from build123d import *

# Parameters (mm, degrees)
SKETCH1_R           = 8.3185
BOSS_EXTRUDE1_DEPTH = 6.35
FILLET1_R           = 0.508
SHELL1_T            = -0.127
SKETCH11_W          = 13.94567027
SKETCH11_H          = 5.377156333
CUT_EXTRUDE1_DEPTH  = 9.144
BOSS_EXTRUDE2_DEPTH = 1.27
SKETCH14_R          = 2.413
SKETCH14_R_2        = 2.316819153
CUT_EXTRUDE2_DEPTH  = 0.0254


with BuildPart() as part:
    # Sketch1 → Boss-Extrude1 (new body)
    with BuildSketch(Plane(origin=(0, 0, 0), x_dir=(1, 0, 0), z_dir=(0, 1, 0))):
        with Locations(Location((0, 0, 0), (0, 0, 270))):
            Circle(SKETCH1_R)
    extrude(amount=BOSS_EXTRUDE1_DEPTH)

    # Fillet1
    fillet1_edges = [part.edges().sort_by_distance(p)[0] for p in [
        (0, 0, -8.3185),
    ]]
    fillet(fillet1_edges, radius=FILLET1_R)

    # Shell1
    shell1_openings = [part.faces().sort_by_distance(p)[0] for p in [
        (0, 6.35, 0),
    ]]
    offset(amount=SHELL1_T, openings=shell1_openings, kind=Kind.INTERSECTION)

    # Sketch11 → Cut-Extrude1 (cut)
    with BuildSketch(Plane.XY):
        with Locations((0, 7.768578167)):
            Rectangle(SKETCH11_W, SKETCH11_H)
    extrude(amount=-CUT_EXTRUDE1_DEPTH, mode=Mode.SUBTRACT)

    # Sketch12 → Boss-Extrude2 (add)
    with BuildSketch(Plane(origin=(0, 6.35, 0), x_dir=(1, 0, 0), z_dir=(0, 1, 0))):
        with BuildLine():
            Line((-7.133425829, 4.026773918), (-7.253796585, 4.071839554))
            ThreePointArc((-7.253796585, 4.071839554), (-7.632439491, 3.308067361), (-7.930925759, 2.509553516))
            Line((-7.930925759, 2.509553516), (-7.811826035, 2.464963741))
            ThreePointArc((-7.811826035, 2.464963741), (-7.513318247, 3.263544265), (-7.133425829, 4.026773918))
        make_face()
        with BuildLine():
            Line((7.811826035, 2.464963741), (7.930925759, 2.509553516))
            ThreePointArc((7.930925759, 2.509553516), (7.632439491, 3.308067361), (7.253796585, 4.071839554))
            Line((7.253796585, 4.071839554), (7.133425829, 4.026773918))
            ThreePointArc((7.133425829, 4.026773918), (7.513318247, 3.263544265), (7.811826035, 2.464963741))
        make_face()
        with BuildLine():
            Line((7.133425829, -4.026773918), (7.253796585, -4.071839554))
            ThreePointArc((7.253796585, -4.071839554), (7.632439491, -3.308067361), (7.930925759, -2.509553516))
            Line((7.930925759, -2.509553516), (7.811826035, -2.464963741))
            ThreePointArc((7.811826035, -2.464963741), (7.513318247, -3.263544265), (7.133425829, -4.026773918))
        make_face()
        with BuildLine():
            Line((-7.811826035, -2.464963741), (-7.930925759, -2.509553516))
            ThreePointArc((-7.930925759, -2.509553516), (-7.632439491, -3.308067361), (-7.253796585, -4.071839554))
            Line((-7.253796585, -4.071839554), (-7.133425829, -4.026773918))
            ThreePointArc((-7.133425829, -4.026773918), (-7.513318247, -3.263544265), (-7.811826035, -2.464963741))
        make_face()
    extrude(amount=BOSS_EXTRUDE2_DEPTH)

    # Sweep1: sweep along a curve in space
    with BuildLine() as sweep1_path:
        ThreePointArc((-7.253796585, 7.62, -4.071839554), (-7.632439491, 7.62, -3.308067361), (-7.930925759, 7.62, -2.509553516))
    # Sketch13 → Sweep1 (sweep)
    with BuildSketch(Plane(origin=(-0.150951504, 0, 0.403192943), x_dir=(0.9365167851453156, 0, 0.35062274760928275), z_dir=(-0.35062274760928275, 0, 0.9365167851453156))):
        with BuildLine():
            Line((-8.180178564, 7.62), (-8.180178564, 7.880813702))
            ThreePointArc((-8.180178564, 7.880813702), (-8.105783687, 8.060418825), (-7.926178564, 8.134813702))
            Line((-7.926178564, 8.134813702), (-6.82245156, 8.134813702))
            Line((-6.82245156, 8.134813702), (-6.82245156, 8.261813702))
            Line((-6.82245156, 8.261813702), (-7.926351644, 8.261813702))
            ThreePointArc((-7.926351644, 8.261813702), (-8.195759328, 8.150221386), (-8.307351644, 7.880813702))
            Line((-8.307351644, 7.880813702), (-8.307351644, 7.62))
            Line((-8.307351644, 7.62), (-8.180178564, 7.62))
        make_face()
    sweep1 = sweep(path=sweep1_path.line)

    # Mirror1: Sweep1 across plane
    add(sweep1.mirror(Plane(origin=(0, 0, 0), x_dir=(0, 0, 1), z_dir=(1, 0, 0))))

    # Mirror2: Sweep1 across plane
    add(sweep1.mirror(Plane.XY))

    # Mirror2 copy 1: sweep along a curve in space
    with BuildLine() as mirror2_copy_1_path:
        ThreePointArc((7.253796585, 7.62, 4.071839554), (7.632439491, 7.62, 3.308067361), (7.930925759, 7.62, 2.509553516))
    # Mirror2 copy 1 sketch → Mirror2 copy 1 (sweep)
    with BuildSketch(Plane(origin=(0.150951504, 0, -0.403192943), x_dir=(-0.9365167851453156, 0, -0.35062274760928275), z_dir=(0.35062274760928275, 0, -0.9365167851453156))):
        with BuildLine():
            Line((-8.180178564, 7.62), (-8.180178564, 7.880813702))
            ThreePointArc((-8.180178564, 7.880813702), (-8.105783687, 8.060418825), (-7.926178564, 8.134813702))
            Line((-7.926178564, 8.134813702), (-6.82245156, 8.134813702))
            Line((-6.82245156, 8.134813702), (-6.82245156, 8.261813702))
            Line((-6.82245156, 8.261813702), (-7.926351644, 8.261813702))
            ThreePointArc((-7.926351644, 8.261813702), (-8.195759328, 8.150221386), (-8.307351644, 7.880813702))
            Line((-8.307351644, 7.880813702), (-8.307351644, 7.62))
            Line((-8.307351644, 7.62), (-8.180178564, 7.62))
        make_face()
    sweep(path=mirror2_copy_1_path.line)

    # Sketch14 → Cut-Extrude2 (cut)
    with BuildSketch(Plane.XZ):
        with Locations(Location((0, 0, 0), (0, 0, 270))):
            Circle(SKETCH14_R)
        with Locations(Location((0, 0, 0), (0, 0, 270))):
            Circle(SKETCH14_R_2, mode=Mode.SUBTRACT)
    extrude(amount=-CUT_EXTRUDE2_DEPTH, mode=Mode.SUBTRACT)


solid = part.part
The model under review builds one solid part; all positions refer to its coordinate system, in mm. Coordinates: 2 decimals unless noted, no trailing zeros. Write each loop counter-clockwise with the first axis right and the second up, starting at its lowest first coordinate (ties: lowest second). Pieces come first, ordered by that corner, then holes. Notation, with made-up numbers: (-5.75, 62) - (43.25, 62) arc R19 ccw to (43.25, 88) - close; hole circle Ø6 at (36, -38.5). An arc over 180 degrees is marked (long way). Answer as a JSON object with one key per item and string values. Group by question number.
1. Add section D-D (y = 5.5). Give the boundary of the cut face in (x, z), plus the area to 3 significant figures.
2. Clearance check with flat-ended pins moving along their axes: pin 1 Ø2 at (x, z) = (-1, -4) entering from +Y; pin 2 Ø3 at (y, z) = (3.5, 2) entering from -X; pin 3 Ø2 at (x, y) = (6, 7) entering from -Z. State where each tip first meets the part, or that it passes through.
3. To check wall thickness, follow probe 1 along Z at (x, y) = (-7.5, 5); probe 2 along Z at (x, y) = (6, 3.25); probe 3 along X at (y, z) = (4.75, -5.5). State the ranges of each line that lie inside material, in increasing order.
4. Add section B-B (y = 1.5). Give the boundary of the cut face in (x, z).
Findings:
{
 "1": {"outline": "(-6.97, -4.54) - (-6.97, -4.3) arc R8.19 cw (long way) to (6.97, -4.3) - (6.97, -4.54) arc R8.32 ccw (long way) to start", "area": "4.48 mm²"},
 "2": {"pin 1": "y = 0.13", "pin 2": "x = -8.3", "pin 3": "z = 4.63"},
 "3": {"probe 1": "-3.6 to -3.29, 3.29 to 3.6", "probe 2": "-5.76 to -5.58, 5.58 to 5.76", "probe 3": "-6.24 to -6.07, 6.07 to 6.24"},
 "4": {"outline": "circle Ø16.64 at (0, 0); hole circle Ø16.38 at (0, 0)"}
}
